Build history of the part. All positions in model axes, mm. Face numbers are marked on the shaded views. A direction names the side the tool comes from. Coordinates: 2 decimals unless noted, no trailing zeros. Loops run counter-clockwise (first coordinate to the right, second up) from the corner with the lowest first, then second, coordinate; pieces in that order, holes last.
Item 1: Cut at C-C (z = -6.5). List the corners of the cut face in (x, y), and give its area (3 significant figures).
Item 2: Mould opens along Y. For the marked faces 5, 6 and 7 say: released by +Y, released by -Y, zero draft, split by the parting line, or undercut.
Item 3: Flat gauge pins, fed straight in: pin 1 (3.5 mm diameter, centred on x = 6, z = -4.5, fed in from -Y); pin 2 (1 mm diameter, centred on y = -1.5, z = -2, fed in from -X); pin 3 (0.8 mm diameter, centred on y = 9, z = -2.5, fed in from -X). Where does each tip first touch, or does it go through?
Item 4: Cut at A-A (x = 25). List the corners of the cut face in (y, z), and give its area (3 significant figures).
Item 5: Drill centre lines: line 1 along X through (y, z) = (3.1, -5); line 2 along X through (y, z) = (3.75, -5); line 3 along X through (y, z) = (-12.5, -1.5). Where is each one in solid material? Low to high.
Item 6: 3-axis set-ups, long thin cutter, end or side, ignore diameter. For the marked faces 1, 2, 3 and 4: which of +Z, -Z, +X, -X, +Y, -Y reach the whole face in a straight line?
Item 7: Cut at B-B (y = -10). List the corners of the cut face in (x, z), and give its area (3 significant figures).
from build123d import *

# Parameters (mm, degrees)
BOSS_EXTRUDE1_DEPTH     = 10
SKETCH2_W               = 11.5
SKETCH2_H               = 17.246462599
CUT_EXTRUDE1_DEPTH      = 2
FILLET1_R               = 5
SKETCH4_R               = 2.15
CUT_EXTRUDE4_DEPTH      = 5
SKETCH6_W               = 10
SKETCH6_H               = 10
BOSS_EXTRUDE2_DEPTH     = 15
SKETCH5_R               = 2
CUT_EXTRUDE5_DEPTH      = 7
SKETCH7_W               = 8.5
SKETCH7_H               = 10
CUT_EXTRUDE6_DEPTH      = 0.5
CUT_EXTRUDE7_DEPTH      = 36
CUT_EXTRUDE7_DEPTH_BACK = 36
SKETCH8_R               = 2
FILLET2_R               = 3


with BuildPart() as part:
    # Sketch1 → Boss-Extrude1 (new body)
    with BuildSketch(Plane(origin=(0, 0, 0), x_dir=(1, 0, 0), z_dir=(0, 1, 0))):
        Polygon((0, 0), (20, 0), (30, 0), (30, 10), (0, 10), align=None)
    extrude(amount=BOSS_EXTRUDE1_DEPTH)

    # Sketch2 → Cut-Extrude1 (cut)
    with BuildSketch(Plane(origin=(0, 10, 0), x_dir=(1, 0, 0), z_dir=(0, 1, 0))):
        with Locations((15.75, 1.3767687)):
            Rectangle(SKETCH2_W, SKETCH2_H)
    extrude(amount=-CUT_EXTRUDE1_DEPTH, mode=Mode.SUBTRACT)

    # Fillet1
    fillet1_edges = [part.edges().sort_by_distance(p)[0] for p in [
        (0, 5, -10),
        (0, 5, 0),
    ]]
    fillet(fillet1_edges, radius=FILLET1_R - 0.0001)  # a hair under: the kernel refuses the full size

    # Sketch4 → Cut-Extrude4 (cut)
    with BuildSketch(Plane.XZ):
        with Locations(Location((6.5, -5, 0), (0, 0, 270))):
            Circle(SKETCH4_R)
    extrude(amount=-CUT_EXTRUDE4_DEPTH, mode=Mode.SUBTRACT)

    # Sketch6 → Boss-Extrude2 (add)
    with BuildSketch(Plane.XZ):
        with Locations((25, -5)):
            Rectangle(SKETCH6_W, SKETCH6_H)
    extrude(amount=BOSS_EXTRUDE2_DEPTH)

    # Sketch5 → Cut-Extrude5 (cut)
    with BuildSketch(Plane.XY):
        with Locations((25, 3)):
            Circle(SKETCH5_R)
        with Locations((25, -10)):
            Circle(SKETCH5_R)
    extrude(amount=-CUT_EXTRUDE5_DEPTH, mode=Mode.SUBTRACT)

    # Sketch7 → Cut-Extrude6 (cut)
    with BuildSketch(Plane(origin=(0, 10, 0), x_dir=(1, 0, 0), z_dir=(0, 1, 0))):
        with Locations((25.75, 5)):
            Rectangle(SKETCH7_W, SKETCH7_H)
    extrude(amount=-CUT_EXTRUDE6_DEPTH, mode=Mode.SUBTRACT)

    # Sketch8 → Cut-Extrude7 (cut, two sides: drawn at the far end of the back side and taken through both)
    with BuildSketch(Plane(origin=(0, 0, -10), x_dir=(-1, 0, 0), z_dir=(0, 0, -1)).offset(-CUT_EXTRUDE7_DEPTH_BACK)):
        with Locations((-20, -2)):
            Circle(SKETCH8_R)
    extrude(amount=CUT_EXTRUDE7_DEPTH + CUT_EXTRUDE7_DEPTH_BACK, mode=Mode.SUBTRACT)

    # Fillet2
    fillet2_edges = [part.edges().sort_by_distance(p)[0] for p in [
        (20, -4, -5),
    ]]
    fillet(fillet2_edges, radius=FILLET2_R)


solid = part.part
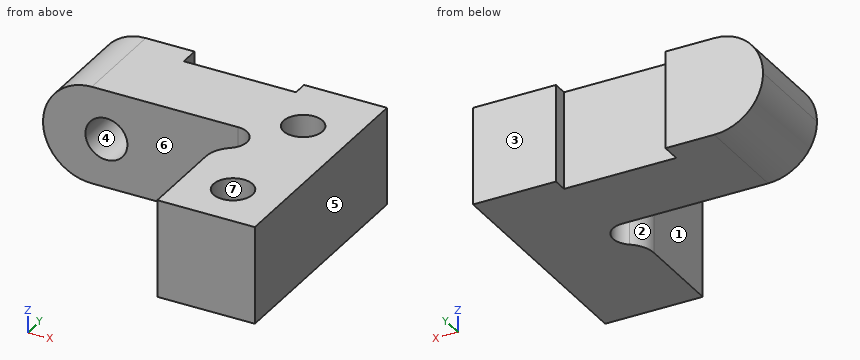
Filled sheet:
1. outline: (0.23, 0) - (4.96, 0) - (4.96, 5) - (8.04, 5) - (8.04, 0) - (20, 0) arc R2 cw to (21.2, -3.6) arc R3 ccw to (20, -6) - (20, -15) - (30, -15) - (30, 9.5) - (21.5, 9.5) - (21.5, 8) - (10, 8) - (10, 10) - (0.23, 10) - close; hole circle Ø4 at (25, -10); hole circle Ø4 at (25, 3)
1. area: 373 mm2
2. face 5: zero draft
2. face 6: released by -Y
2. face 7: undercut
3. pin 1: stops at y = 0
3. pin 2: stops at x = 21.73
3. pin 3: stops at x = 0.46
4. outline: (-15, -10) - (9.5, -10) - (9.5, 0) - (5, 0) - (5, -7) - (1, -7) - (1, 0) - (-8, 0) - (-8, -7) - (-12, -7) - (-12, 0) - (-15, 0) - close
4. area: 189 mm2
5. line 1: x = 0 to 4.35, 8.65 to 23, 27 to 30
5. line 2: x = 0 to 4.35, 8.65 to 23.15, 26.85 to 30
5. line 3: x = 20 to 30
6. face 1: +Z, -Z, -X, -Y
6. face 2: +Z, -Z, -X
6. face 3: +Z, -Z, +X, +Y
6. face 4: -Y
7. outline: (20, -10) - (30, -10) - (30, 0) - (27, 0) - (27, -7) - (23, -7) - (23, 0) - (20, 0) - close
7. area: 72.0 mm2
